Model file for the job. Use its own axes, mm. Face numbers are marked on the shaded views. A direction names the side the tool comes from. Round coordinates to 2 decimals unless told otherwise and drop trailing zeros. Loops run counter-clockwise (first coordinate to the right, second up) from the corner with the lowest first, then second, coordinate; pieces in that order, holes last. Notation, with made-up numbers: M -25,3.25 L 10,3.25 A22 cw 10,30.25 Z; hole C 57,14.5 d8. An arc over 180 degrees is marked long. Use a Markdown table: item, result. Add a question column.
Q1. Cut at B-B (y = -8.5). Give the cut face in (x, z).
Q2. Tool access for the marked faces 4, 5 and 6: list every direction of +Z, -Z, +X, -X, +Y, -Y with a clear straight run to the whole face (end or side of a thin tool).
Q3. Pin check, flat tips, straight feed: pin 1 (12 mm diameter, centred on y = 14.5, z = 4, fed in from +X); pin 2 (4 mm diameter, centred on x = -7, z = -4, fed in from +Y); pin 3 (10 mm diameter, centred on x = -2, y = 6.5, fed in from +Z); pin 4 (1.5 mm diameter, centred on x = 6, y = 6.5, fed in from +Z). Stop position of each tip, or through.
Q4. Mould opens along Z. For the marked faces 1, 2 and 3 say: +Z half, -Z half, draft (parallel to the pull), parting line (faces both ways), or undercut.
Q5. Cut at D-D (z = -7.5). Give the cut face in (x, y), plus the area to 3 significant figures.
Q6. Cut at A-A (y = 7.5). Give the cut face in (x, z).
Q7. Cut at C-C (x = 8.5). Give the cut face in (y, z), plus the area to 3 significant figures.
Q8. Probe line 1 (Z direction, x = 0, y = -7.25); line 2 (Y direction, x = -6, z = -5.5); line 3 (Y direction, x = -3.75, z = 5). List the from-to ranges inside material, lowest first. Write a range as from..to.
from build123d import *

# Parameters (mm, degrees)
F0_R      = 10.16
F1_DEPTH  = 5.08
F2_R      = 6.35
F2_R_2    = 5.08
F3_DEPTH  = 10.16
F4_R      = 6.35
F5_DEPTH  = 5.08
F6_R      = 5.08
F7_DEPTH  = 5.08
F8_R      = 3.81
F9_DEPTH  = 5.08
F10_R     = 2.54
F11_DEPTH = 5.08
F12_R     = 1.27
F13_DEPTH = 5.08
F14_R     = 0.635
F15_DEPTH = 5.08


with BuildPart() as f1:
    # F0 (on Front) → F1 (new body)
    with BuildSketch(Plane.XZ):
        Circle(F0_R)
    extrude(amount=F1_DEPTH)

    # F2 (on face) → F3 (join)
    with BuildSketch(Plane.XZ.offset(5.08)):
        Circle(F2_R)
        Circle(F2_R_2, mode=Mode.SUBTRACT)
    extrude(amount=F3_DEPTH)

    # F4 (on face) → F5 (join)
    with BuildSketch(Plane(origin=(0, 0, 0), x_dir=(-1, 0, 0), z_dir=(0, 1, 0))):
        Circle(F4_R)
    extrude(amount=F5_DEPTH)

    # F6 (on face) → F7 (join)
    with BuildSketch(Plane(origin=(0, 5.08, 0), x_dir=(-1, 0, 0), z_dir=(0, 1, 0))):
        Circle(F6_R)
    extrude(amount=F7_DEPTH)

    # F8 (on face) → F9 (join)
    with BuildSketch(Plane(origin=(0, 10.16, 0), x_dir=(-1, 0, 0), z_dir=(0, 1, 0))):
        Circle(F8_R)
    extrude(amount=F9_DEPTH)

    # F10 (on face) → F11 (join)
    with BuildSketch(Plane(origin=(0, 15.24, 0), x_dir=(-1, 0, 0), z_dir=(0, 1, 0))):
        Circle(F10_R)
    extrude(amount=F11_DEPTH)

    # F12 (on face) → F13 (join)
    with BuildSketch(Plane(origin=(0, 20.32, 0), x_dir=(-1, 0, 0), z_dir=(0, 1, 0))):
        Circle(F12_R)
    extrude(amount=F13_DEPTH)

    # F14 (on face) → F15 (join)
    with BuildSketch(Plane(origin=(0, 25.4, 0), x_dir=(-1, 0, 0), z_dir=(0, 1, 0))):
        Circle(F14_R)
    extrude(amount=F15_DEPTH)


solid = f1.part
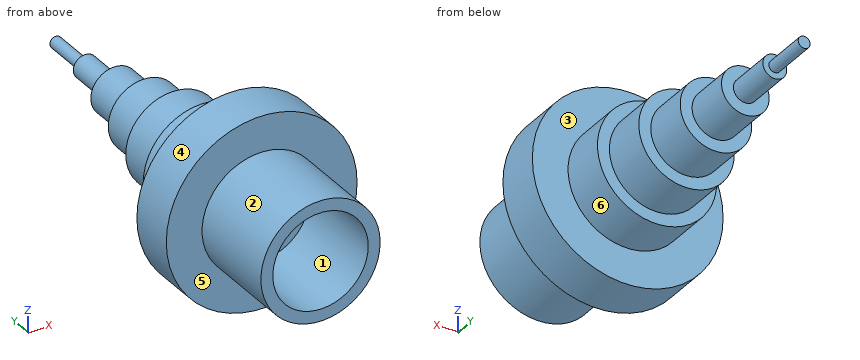
Checked values:
| question | item | result |
|---|---|---|
| 1 | outline | C 0,0 d12.7; hole C 0,0 d10.16 |
| 2 | face 4 | +Y, -Y |
| 2 | face 5 | -Y |
| 2 | face 6 | +Y |
| 3 | pin 1 | stops at x = 5.08 |
| 3 | pin 2 | stops at y = 5.08 |
| 3 | pin 3 | stops at z = 6.35 |
| 3 | pin 4 | passes through |
| 4 | face 1 | undercut |
| 4 | face 2 | parting line |
| 4 | face 3 | draft |
| 5 | outline | M -6.85,-5.08 L 6.85,-5.08 L 6.85,0 L -6.85,0 Z |
| 5 | area | 69.6 mm^2 |
| 6 | outline | C 0,0 d10.16 |
| 7 | outline | M -5.08,-5.57 L 0,-5.57 L 0,5.57 L -5.08,5.57 Z |
| 7 | area | 56.5 mm^2 |
| 8 | line 1 | z = -6.35..-5.08, 5.08..6.35 |
| 8 | line 2 | y = -5.08..0 |
| 8 | line 3 | y = -15.24..5.08 |
